Here's how the part is built. I have some questions about the finished solid (model axes, mm). Coordinates: 2 decimals unless noted, no trailing zeros. Write each loop counter-clockwise with the first axis right and the second up, starting at its lowest first coordinate (ties: lowest second). Pieces come first, ordered by that corner, then holes.
Item 1: If we section it at B-B (y = 1.1): Count the separate pieces of the cut face and the enclosed holes in it, then the cut area to 3 significant figures.
Item 2: If I drill on line 1 (Z direction, x = -19.05, y = 1.15); line 2 (Z direction, x = -178.5, y = 0.4); line 3 (X direction, y = 0.55, z = -169.5), over which ranges is the centre line in solid material (lowest first)?
Item 3: If we section it at A-A (x = -135.5): Please give me the cut outline in (y, z), then the cut area to 3 significant figures.
Item 4: I'm going to push flat-ended pins straight in: pin 1 Ø1.3 at (y, z) = (1, -95) entering from +X; pin 2 Ø1.5 at (x, y) = (-91.5, 0.5) entering from -Z; pin 3 Ø1 at (x, y) = (-130, 0.5) entering from +Z. Where does each tip first touch, or does it pass through?
Item 5: If we section it at C-C (z = -315.5): Please give me the cut outline in (x, y), then the cut area to 3 significant figures.
from build123d import *

# Parameters (mm, degrees)
BOSS_EXTRUDE1_DEPTH     = 2.54
FILLET1_R               = 6.35
SKETCH2_W               = 12.954
SKETCH2_H               = 19.304
SKETCH2_W_2             = 12.7
SKETCH2_H_2             = 19.05
CUT_EXTRUDE1_DEPTH      = 498.15765659
F_1_4_CLEARANCE_HOLE1_D = 6.7564
SKETCH5_R               = 0.79375
CUT_EXTRUDE2_DEPTH      = 498.15765659


with BuildPart() as part:
    # Sketch1 → Boss-Extrude1 (new body)
    with BuildSketch(Plane(origin=(0, 0, 0), x_dir=(1, 0, 0), z_dir=(0, 1, 0))):
        Polygon((0, 0), (-80.9625, 0), (-80.9625, 76.2), (-195.2625, 76.2), (-195.2625, 307.35814247), (-80.645, 457.2), (0, 457.2), align=None)
    extrude(amount=BOSS_EXTRUDE1_DEPTH)

    # Fillet1
    fillet1_edges = [part.edges().sort_by_distance(p)[0] for p in [
        (-80.9625, 1.27, -76.2),
        (-195.2625, 1.27, -76.2),
    ]]
    fillet(fillet1_edges, radius=FILLET1_R)

    # Sketch2 → Cut-Extrude1 (cut, through all)
    with BuildSketch(Plane(origin=(0, 2.54, 0), x_dir=(1, 0, 0), z_dir=(0, 1, 0))):
        with Locations((-74.6125, 413.385)):
            Rectangle(SKETCH2_W, SKETCH2_H)
        with Locations((-74.6125, 413.385)):
            Rectangle(SKETCH2_W_2, SKETCH2_H_2, mode=Mode.SUBTRACT)
        with Locations((-188.9125, 288.139828218)):
            Rectangle(SKETCH2_W, SKETCH2_H)
        with Locations((-188.9125, 288.139828218)):
            Rectangle(SKETCH2_W_2, SKETCH2_H_2, mode=Mode.SUBTRACT)
        with Locations((-74.6125, 294.3225)):
            Rectangle(SKETCH2_W, SKETCH2_H)
        with Locations((-74.6125, 294.3225)):
            Rectangle(SKETCH2_W_2, SKETCH2_H_2, mode=Mode.SUBTRACT)
        with Locations((-188.9125, 225.7425)):
            Rectangle(SKETCH2_W, SKETCH2_H)
        with Locations((-188.9125, 225.7425)):
            Rectangle(SKETCH2_W_2, SKETCH2_H_2, mode=Mode.SUBTRACT)
        with Locations((-188.9125, 143.1925)):
            Rectangle(SKETCH2_W, SKETCH2_H)
        with Locations((-188.9125, 143.1925)):
            Rectangle(SKETCH2_W_2, SKETCH2_H_2, mode=Mode.SUBTRACT)
        with Locations((-74.6125, 162.8775)):
            Rectangle(SKETCH2_W, SKETCH2_H)
        with Locations((-74.6125, 162.8775)):
            Rectangle(SKETCH2_W_2, SKETCH2_H_2, mode=Mode.SUBTRACT)
        with Locations((-74.6125, 43.815)):
            Rectangle(SKETCH2_W, SKETCH2_H)
        with Locations((-74.6125, 43.815)):
            Rectangle(SKETCH2_W_2, SKETCH2_H_2, mode=Mode.SUBTRACT)
        with Locations((-6.35, 93.82125)):
            Rectangle(SKETCH2_W, SKETCH2_H)
        with Locations((-6.35, 93.82125)):
            Rectangle(SKETCH2_W_2, SKETCH2_H_2, mode=Mode.SUBTRACT)
        with Locations((-6.35, 171.45)):
            Rectangle(SKETCH2_W, SKETCH2_H)
        with Locations((-6.35, 171.45)):
            Rectangle(SKETCH2_W_2, SKETCH2_H_2, mode=Mode.SUBTRACT)
        with Locations((-6.35, 244.475)):
            Rectangle(SKETCH2_W, SKETCH2_H)
        with Locations((-6.35, 244.475)):
            Rectangle(SKETCH2_W_2, SKETCH2_H_2, mode=Mode.SUBTRACT)
        with Locations((-6.35, 317.5)):
            Rectangle(SKETCH2_W, SKETCH2_H)
        with Locations((-6.35, 317.5)):
            Rectangle(SKETCH2_W_2, SKETCH2_H_2, mode=Mode.SUBTRACT)
        with Locations((-6.35, 390.525)):
            Rectangle(SKETCH2_W, SKETCH2_H)
        with Locations((-6.35, 390.525)):
            Rectangle(SKETCH2_W_2, SKETCH2_H_2, mode=Mode.SUBTRACT)
    extrude(amount=-CUT_EXTRUDE1_DEPTH, mode=Mode.SUBTRACT)


with BuildPart() as cut_extrude1_kept_piece:
    # of the separate pieces the step leaves, the one the design keeps (cut_extrude1_pieces_kept)
    add(part.part.solids().sort_by_distance((-80.9625, 0, -34.163))[0])

    # 1/4 Clearance Hole1 (through all)
    with Locations(Plane(origin=(0, 0, 0), x_dir=(-1, 0, 0), z_dir=(0, -1, 0))):
        with Locations((61.9125, 97.155), (19.05, 134.9375), (19.05, 207.9625), (61.9125, 228.6), (19.05, 280.9875), (19.05, 354.0125), (61.9125, 360.045), (19.05, 427.0375), (176.2125, 259.08), (176.2125, 192.405), (176.2125, 93.98)):
            Hole(F_1_4_CLEARANCE_HOLE1_D / 2)

    # Sketch5 → Cut-Extrude2 (cut, through all)
    with BuildSketch(Plane(origin=(0, 2.54, 0), x_dir=(1, 0, 0), z_dir=(0, 1, 0))):
        with Locations((-182.4355, 296.998078218)):
            Circle(SKETCH5_R)
        with Locations((-182.4355, 279.281578218)):
            Circle(SKETCH5_R)
        with Locations((-182.4355, 234.60075)):
            Circle(SKETCH5_R)
        with Locations((-182.4355, 216.88425)):
            Circle(SKETCH5_R)
        with Locations((-182.4355, 152.05075)):
            Circle(SKETCH5_R)
        with Locations((-182.4355, 134.33425)):
            Circle(SKETCH5_R)
        with Locations((-68.1355, 52.67325)):
            Circle(SKETCH5_R)
        with Locations((-68.1355, 34.95675)):
            Circle(SKETCH5_R)
        with Locations((-12.827, 84.963)):
            Circle(SKETCH5_R)
        with Locations((-12.827, 102.6795)):
            Circle(SKETCH5_R)
        with Locations((-68.1355, 171.73575)):
            Circle(SKETCH5_R)
        with Locations((-81.0895, 171.73575)):
            Circle(SKETCH5_R)
        with Locations((-81.0895, 154.01925)):
            Circle(SKETCH5_R)
        with Locations((-68.1355, 154.01925)):
            Circle(SKETCH5_R)
        with Locations((-12.827, 162.59175)):
            Circle(SKETCH5_R)
        with Locations((-12.827, 180.30825)):
            Circle(SKETCH5_R)
        with Locations((-12.827, 235.61675)):
            Circle(SKETCH5_R)
        with Locations((-12.827, 253.33325)):
            Circle(SKETCH5_R)
        with Locations((-68.1355, 285.46425)):
            Circle(SKETCH5_R)
        with Locations((-81.0895, 285.46425)):
            Circle(SKETCH5_R)
        with Locations((-81.0895, 303.18075)):
            Circle(SKETCH5_R)
        with Locations((-68.1355, 303.18075)):
            Circle(SKETCH5_R)
        with Locations((-12.827, 308.64175)):
            Circle(SKETCH5_R)
        with Locations((-12.827, 326.35825)):
            Circle(SKETCH5_R)
        with Locations((-12.827, 399.38325)):
            Circle(SKETCH5_R)
        with Locations((-12.827, 381.66675)):
            Circle(SKETCH5_R)
        with Locations((-68.1355, 422.24325)):
            Circle(SKETCH5_R)
        with Locations((-81.0895, 422.24325)):
            Circle(SKETCH5_R)
        with Locations((-81.0895, 404.52675)):
            Circle(SKETCH5_R)
        with Locations((-68.1355, 404.52675)):
            Circle(SKETCH5_R)
    extrude(amount=-CUT_EXTRUDE2_DEPTH, mode=Mode.SUBTRACT)


solid = cut_extrude1_kept_piece.part
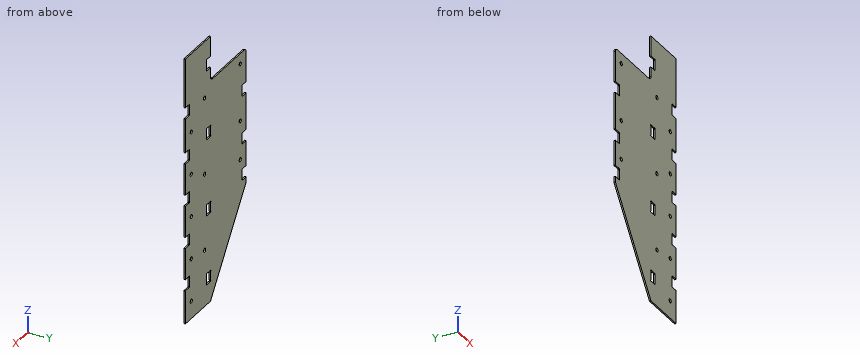
Answer list:
1. separate pieces: 1
1. enclosed holes: 14
1. area: 68,600 mm2
2. line 1: z = -457.2 to -430.42, -423.66 to -357.39, -350.63 to -284.37, -277.61 to -211.34, -204.58 to -138.32, -131.56 to 0
2. line 2: z = -329.27 to -261.57, -256.59 to -194.89, -189.92 to -96.47, -91.49 to -76.2
2. line 3: x = -195.26 to -81.09, -68.14 to -12.83
3. outline: (0, -385.49) - (2.54, -385.49) - (2.54, -76.2) - (0, -76.2) - close
3. area: 786 mm2
4. pin 1: stops at x = -12.83
4. pin 2: stops at z = -443.99
4. pin 3: stops at z = -76.2
5. outline: (-189.03, 0) - (-12.83, 0) - (-12.83, 2.54) - (-189.03, 2.54) - close
5. area: 448 mm2
